from build123d import *

# Parameters (mm, degrees)
SKETCH1_R           = 40
BOSS_EXTRUDE1_DEPTH = 10
SKETCH12_R          = 15
BOSS_EXTRUDE3_DEPTH = 10
SKETCH13_R          = 7.5
BOSS_EXTRUDE4_DEPTH = 95
CUT_EXTRUDE1_DEPTH  = 120.268604419
SKETCH17_R          = 2.5
CUT_EXTRUDE3_DEPTH  = 120.268604507
SKETCH18_R          = 1.5
CUT_EXTRUDE4_DEPTH  = 120.268604507


with BuildPart() as part:
    # Sketch1 → Boss-Extrude1 (new body)
    with BuildSketch(Plane.XY):
        Circle(SKETCH1_R)
    extrude(amount=BOSS_EXTRUDE1_DEPTH)

    # Sketch12 → Boss-Extrude3 (add)
    with BuildSketch(Plane(origin=(0, 0, 0), x_dir=(-1, 0, 0), z_dir=(0, 0, -1))):
        with Locations(Location((0, 0, 0), (0, 0, 180))):
            Circle(SKETCH12_R)
    extrude(amount=BOSS_EXTRUDE3_DEPTH)

    # Sketch13 → Boss-Extrude4 (add)
    with BuildSketch(Plane.XY.offset(10)):
        Circle(SKETCH13_R)
    extrude(amount=BOSS_EXTRUDE4_DEPTH)

    # Sketch14 → Cut-Extrude1 (cut, through all)
    with BuildSketch(Plane(origin=(0, 0, 0), x_dir=(1, 0, 0), z_dir=(0, 1, 0))):
        with BuildLine():
            Line((-2.5, -105), (2.5, -105))
            Line((2.5, -105), (2.5, -96.5))
            ThreePointArc((2.5, -96.5), (0, -94), (-2.5, -96.5))
            Line((-2.5, -96.5), (-2.5, -105))
        make_face()
    cut_extrude1 = extrude(amount=CUT_EXTRUDE1_DEPTH, mode=Mode.SUBTRACT)

    # Mirror4: Cut-Extrude1 across plane
    add(cut_extrude1.mirror(Plane.ZX), mode=Mode.SUBTRACT)

    # Sketch17 → Cut-Extrude3 (cut, through all)
    with BuildSketch(Plane(origin=(0, 0, 0), x_dir=(0, 0, -1), z_dir=(1, 0, 0))):
        with Locations((-101.25, 0)):
            Circle(SKETCH17_R)
    cut_extrude3 = extrude(amount=-CUT_EXTRUDE3_DEPTH, mode=Mode.SUBTRACT)

    # Mirror6: Cut-Extrude3 across plane
    add(cut_extrude3.mirror(Plane(origin=(0, 0, 0), x_dir=(0, 0, 1), z_dir=(1, 0, 0))), mode=Mode.SUBTRACT)

    # Sketch18 → Cut-Extrude4 (cut, through all)
    with BuildSketch(Plane(origin=(0, 0, 0), x_dir=(0, 0, -1), z_dir=(1, 0, 0))):
        with Locations((-5, 0)):
            Circle(SKETCH18_R)
    extrude(amount=-CUT_EXTRUDE4_DEPTH, mode=Mode.SUBTRACT)


solid = part.part
Part model, mm, in its own coordinate system. A direction names the side the tool comes from. Give positions to 0.01 mm unless a question says otherwise; leave off trailing zeros. Loops run counter-clockwise (first coordinate to the right, second up) from the corner with the lowest first, then second, coordinate; pieces in that order, holes last.
(1) Band-saw the part on C-C (x = -5). Write the cut outline in (y, z), and give its area (3 significant figures).
Return value:
outline: (-39.69, 0) - (-14.14, 0) - (-14.14, -10) - (14.14, -10) - (14.14, 0) - (39.69, 0) - (39.69, 10) - (5.59, 10) - (5.59, 105) - (-5.59, 105) - (-5.59, 10) - (-39.69, 10) - close; hole circle Ø5 at (0, 101.25); hole circle Ø3 at (0, 5)
area: 2,110 mm2
(2) Drill centre lines: line 1 along Z through (x, y) = (6.25, 0); line 2 along Z through (x, y) = (21.5, -1.5); line 3 along Y through (x, z) = (-9, 5). Where is each one in solid material? Low to high.
Return value:
line 1: z = -10 to 98.75, 103.75 to 105
line 2: z = 0 to 10
line 3: y = -38.97 to -1.5, 1.5 to 38.97
(3) Band-saw the part on D-D (z = 16). Write the cut outline in (x, y), and give its area (3 significant figures).
Return value:
outline: circle Ø15 at (0, 0)
area: 177 mm2
(4) Pin check, flat tips, straight feed: pin 1 (8 mm diameter, centred on x = 1.5, z = 20.5, fed in from +Y); pin 2 (8 mm diameter, centred on y = 0, z = 101.25, fed in from +X); pin 3 (5 mm diameter, centred on x = 6, y = -31.5, fed in from -Z); pin 4 (4.5 mm diameter, centred on y = 0, z = 101.25, fed in from +X). Stop position of each tip, or through.
Return value:
pin 1: stops at y = 7.5
pin 2: stops at x = 7.5
pin 3: stops at z = 0
pin 4: passes through
(5) 3-axis set-ups, long thin cutter, end or side, ignore diameter. For faces 1 (the cylindrical face through (-19.7, -0.9, 6.2)), 2 (the flat face through (-2.5, 2, 99)), 3 (the cylindrical face through (6.93, -2.87, 56.84)), 4 (the flat face through (-1, -17, 0)): which of +Z, -Z, +X, -X, +Y, -Y reach the whole face in a straight line?
Return value:
face 1: -X
face 2: +Z, +Y, -Y
face 3: +Z
face 4: -Z
(6) Band-saw the part on A-A (y = 0). Write the cut outline in (x, z), and give its area (3 significant figures).
Return value:
outline: (-40, 0) - (-15, 0) - (-15, -10) - (15, -10) - (15, 0) - (40, 0) - (40, 10) - (7.5, 10) - (7.5, 98.75) - (2.5, 98.75) - (2.5, 96.5) arc R2.5 cw to (-2.5, 96.5) - (-2.5, 98.75) - (-7.5, 98.75) - (-7.5, 10) - (-40, 10) - (-40, 6.5) - (0, 6.5) - (0, 3.5) - (-40, 3.5) - close; (-7.5, 103.75) - (-2.5, 103.75) - (-2.5, 105) - (-7.5, 105) - close; (2.5, 103.75) - (7.5, 103.75) - (7.5, 105) - (2.5, 105) - close
area: 2,300 mm2
(7) Band-saw the part on B-B (z = 101.25). Write the cut outline in (x, y), and give its area (3 significant figures).
Return value:
outline: (-7.07, -2.5) arc R7.5 ccw to (-2.5, -7.07) - (-2.5, -2.5) - close; (-7.07, 2.5) - (-2.5, 2.5) - (-2.5, 7.07) arc R7.5 ccw to start; (2.5, -7.07) arc R7.5 ccw to (7.07, -2.5) - (2.5, -2.5) - close; (2.5, 2.5) - (7.07, 2.5) arc R7.5 ccw to (2.5, 7.07) - close
area: 54.5 mm2
(8) Pull direction X, two halves, no side cores. Call faces 5 (the cylindrical face through (8.06, -12.65, -4.93)), 6 (the flat face through (0, 0, 5)), 7 (the flat face through (-4, 0, 105)), 8 (the flat face through (2.5, 2, 99)): pulls with the +X half, pulls with the -X half, needs draft (parallel to the pull), parting line crosses it, or undercut.
Return value:
face 5: parting line crosses it
face 6: pulls with the -X half
face 7: needs draft
face 8: undercut
